Here's the drawing with two shaded views (mm, measured from the low corner). I have some questions. Give positions to 0.01 mm unless a question says otherwise; leave off trailing zeros. Write each loop counter-clockwise with the first axis right and the second up, starting at its lowest first coordinate (ties: lowest second). Pieces come first, ordered by that corner, then holes. Notation, with made-up numbers: (-25.5, -11) - (11.5, -11) arc R30 cw to (11.5, 12) - close; hole circle Ø5 at (-30, -24.75). An arc over 180 degrees is marked (long way). Answer as a JSON object with one key per item and string values. Group by question number.
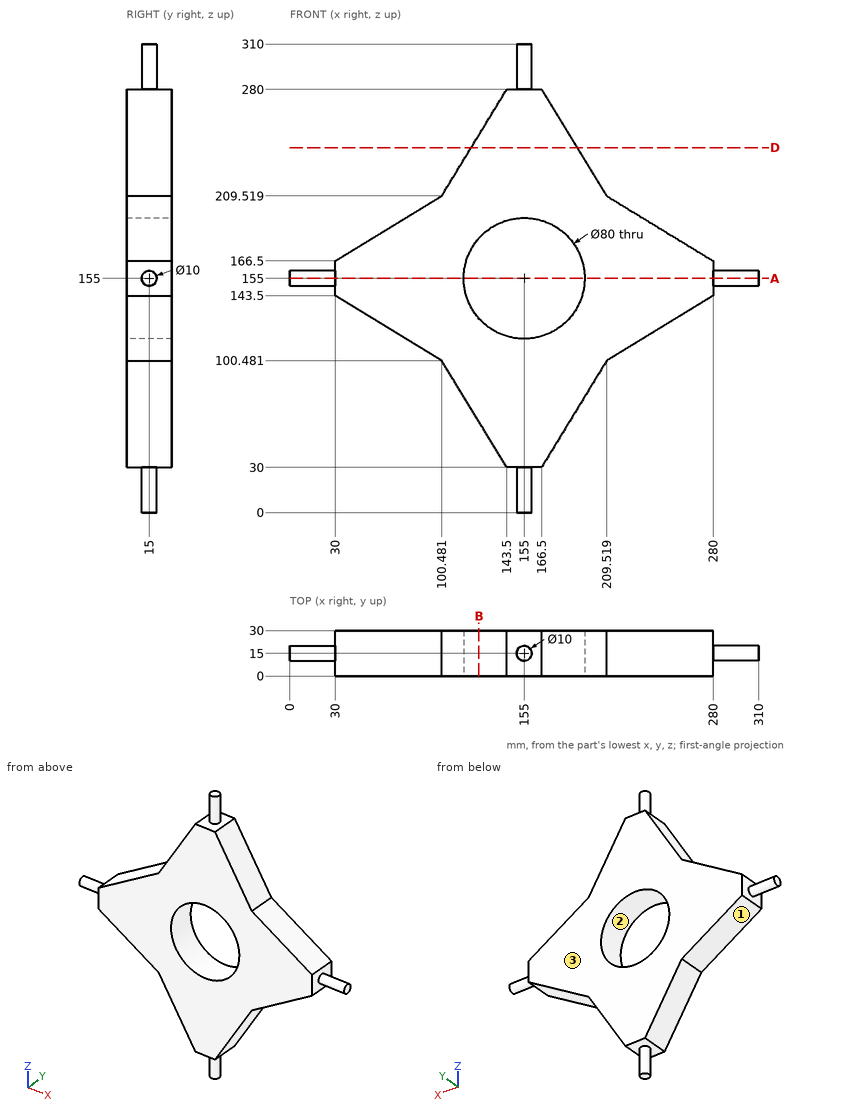
(1) I need wall thicknesses on L1, parallel to X at y = 7, z = 155; L2, parallel to X at y = 19, z = 155; L3, parallel to Z at x = 124.5, y = 17.25. Which ranges of each line are inside material? Lowest first, please.
(2) I want a section at A-A, the plane z = 155. Please give me the cut outline in (x, y).
(3) If we mould it in two halves opening along Z, with no side actions, what happens to the marked faces 1, 2 and 3? For each: +Z half, -Z half, draft (parallel to the pull), parting line (faces both ways), or undercut.
(4) I want a section at D-D, the plane z = 241.5. Please give me the cut outline in (x, y).
(5) Will these pins go through, and if not, where does the flat tip stop? P1, Ø8, axis at y = 21.5, z = 114.5, coming from the +X side; P2, Ø1.5, axis at y = 10.5, z = 180, coming from the -X side; P3, Ø3, axis at y = 23.5, z = 143, coming from the +X side.
(6) I want a section at B-B, the plane x = 125. Please give me the cut outline in (y, z), and give its area (3 significant figures).
Entries:
{
 "1": {"L1": "30 to 115, 195 to 280", "L2": "0 to 115, 195 to 310", "L3": "61.13 to 129.12, 180.88 to 248.87"},
 "2": {"outline": "(0, 10) - (30, 10) - (30, 0) - (115, 0) - (115, 30) - (30, 30) - (30, 20) - (0, 20) - close; (195, 0) - (280, 0) - (280, 10) - (310, 10) - (310, 20) - (280, 20) - (280, 30) - (195, 30) - close"},
 "3": {"face 1": "-Z half", "face 2": "undercut", "face 3": "draft"},
 "4": {"outline": "(120, 0) - (190, 0) - (190, 30) - (120, 30) - close"},
 "5": {"P1": "x = 239.04", "P2": "x = 50.89", "P3": "x = 280"},
 "6": {"outline": "(0, 60.31) - (30, 60.31) - (30, 128.54) - (0, 128.54) - close; (0, 181.46) - (30, 181.46) - (30, 249.69) - (0, 249.69) - close", "area": "4,090 mm^2"}
}
